from build123d import *

# Parameters (mm, degrees)
F0_R      = 15.4644174612
F1_DEPTH  = 7.5
F3_DEPTH  = 3.5
F5_DEPTH  = 7.5
F7_DEPTH  = 7.5
F9_DEPTH  = 7.5
F11_DEPTH = 7.5
F13_DEPTH = 7.5
F15_DEPTH = 7.5
F17_DEPTH = 7.5
F18_W     = 5.4945703596
F18_H     = 28.8444776088
F19_DEPTH = 7.5
F22_DEPTH = 7.5


with BuildPart() as f1:
    # F0 (on Front) → F1 (new body)
    with BuildSketch(Plane.XZ):
        Circle(F0_R)
    extrude(amount=-F1_DEPTH)

    # F2 (on Front) → F3 (join)
    with BuildSketch(Plane.XZ):
        Polygon((3.5883630626, 11.3469837233), (-3.3943967428, 11.3469837233), (-3.3943967428, 3.5883623641), (-10.7650868595, 3.5883623641), (-10.7650868595, -3.5883623641), (-3.3943967428, -3.5883623641), (-3.3943967428, -11.9288796559), (3.5883630626, -11.9288796559), (3.5883630626, -3.5883623641), (11.5409484133, -3.5883623641), (11.5409484133, 3.5883623641), (3.5883630626, 3.5883623641), align=None)
    extrude(amount=F3_DEPTH)

    # F4 (on face) → F5 (join)
    with BuildSketch(Plane.XZ):
        with BuildLine():
            Line((-40.2478465542, -5.0589637569), (-14.6135243224, -5.0589637569))
            ThreePointArc((-14.6135243224, -5.0589637569), (-15.4624028659, 0.2496097512), (-14.442618561, 5.5280174129))
            Line((-14.442618561, 5.5280174129), (-40.2478465542, 5.5280174129))
            Line((-40.2478465542, 5.5280174129), (-40.2478465542, -5.0589637569))
        make_face()
    extrude(amount=-F5_DEPTH)

    # F6 (on face) → F7 (join)
    with BuildSketch(Plane.XZ):
        with BuildLine():
            Line((39.8599132895, 5.5280174129), (14.442618561, 5.5280174129))
            ThreePointArc((14.442618561, 5.5280174129), (15.4559066, 0.512989853), (14.7773852023, -4.5581897721))
            Line((14.7773852023, -4.5581897721), (39.8599132895, -4.5581897721))
            Line((39.8599132895, -4.5581897721), (39.8599132895, 5.5280174129))
        make_face()
    extrude(amount=-F7_DEPTH)

    # F8 (on face) → F9 (join)
    with BuildSketch(Plane.XZ):
        with BuildLine():
            ThreePointArc((13.3392752441, -7.8238061951), (-0.2412620254, -15.4625353694), (-13.5768721894, -7.4038333969))
            Line((-13.5768721894, -7.4038333969), (0, -38.1142273545))
            Line((0, -38.1142273545), (13.3392752441, -7.8238061951))
        make_face()
    extrude(amount=-F9_DEPTH)

    # F10 (on face) → F11 (join)
    with BuildSketch(Plane.XZ):
        with BuildLine():
            Line((1.4583327306, 20.6556674093), (-1.6825530911, 20.6556674093))
            Line((-1.6825530911, 20.6556674093), (-1.6825530911, 15.3955017152))
            Line((-1.6825530911, 15.3955017152), (-1.4583327306, 15.3955017152))
            ThreePointArc((-1.4583327306, 15.3955017152), (0, 15.4644174612), (1.4583327306, 15.3955017152))
            Line((1.4583327306, 15.3955017152), (1.4583327306, 20.6556674093))
        make_face()
    extrude(amount=-F11_DEPTH)

    # F12 (on face) → F13 (join)
    with BuildSketch(Plane.XZ):
        with BuildLine():
            ThreePointArc((1.4583327306, 15.4214656697), (4.3270974304, 17.3693579241), (5.4335625702, 20.6556674093))
            ThreePointArc((5.4335625702, 20.6556674093), (-3.1922832508, 25.05259018), (-1.6825530911, 15.4891775661))
            Line((-1.6825530911, 15.4891775661), (-1.6825530911, 20.6556674093))
            Line((-1.6825530911, 20.6556674093), (1.4583327306, 20.6556674093))
            Line((1.4583327306, 20.6556674093), (1.4583327306, 15.4214656697))
        make_face()
    extrude(amount=-F13_DEPTH)

    # F14 (on face) → F15 (join)
    with BuildSketch(Plane.XZ):
        with BuildLine():
            Line((35.3987067938, 27.0581915975), (2.0601032187, 15.6277874452))
            ThreePointArc((2.0601032187, 15.6277874452), (1.7622400662, 15.5158121435), (1.4583327306, 15.4214656697))
            Line((1.4583327306, 15.4214656697), (1.4583327306, 15.3955017152))
            ThreePointArc((1.4583327306, 15.3955017152), (9.3569158706, 12.312446256), (14.442618561, 5.5280174129))
            Line((14.442618561, 5.5280174129), (35.3987067938, 27.0581915975))
        make_face()
    extrude(amount=-F15_DEPTH)

    # F16 (on face) → F17 (join)
    with BuildSketch(Plane.XZ):
        with BuildLine():
            Line((-1.6825530911, 15.3955017152), (-1.6825530911, 15.4891775661))
            Line((-1.6825530911, 15.4891775661), (-33.5039995381, 25.8523592827))
            Line((-33.5039995381, 25.8523592827), (-14.442618561, 5.5280174129))
            ThreePointArc((-14.442618561, 5.5280174129), (-9.3569158706, 12.312446256), (-1.4583327306, 15.3955017152))
            Line((-1.4583327306, 15.3955017152), (-1.6825530911, 15.3955017152))
        make_face()
    extrude(amount=-F17_DEPTH)

    # F21 (on face) → F22 (join)
    with BuildSketch(Plane.XZ):
        with BuildLine():
            Line((-2.9614820185, 49.562137616), (-2.9614820185, 25.2112383349))
            ThreePointArc((-2.9614820185, 25.2112383349), (-0.8941182921, 26.0151594267), (1.3222555048, 25.9258896612))
            Line((1.3222555048, 25.9258896612), (2.0601032187, 26.0489840022))
            Line((2.0601032187, 26.0489840022), (2.0601032187, 49.562137616))
            Line((2.0601032187, 49.562137616), (-2.9614820185, 49.562137616))
        make_face()
    extrude(amount=-F22_DEPTH)


with BuildPart() as f19:
    # F18 (on Front) → F19 (new body)
    with BuildSketch(Plane.XZ):
        with Locations((0.3433788661, 40.6340872869)):
            Rectangle(F18_W, F18_H)
    extrude(amount=-F19_DEPTH)


solid = f1.part
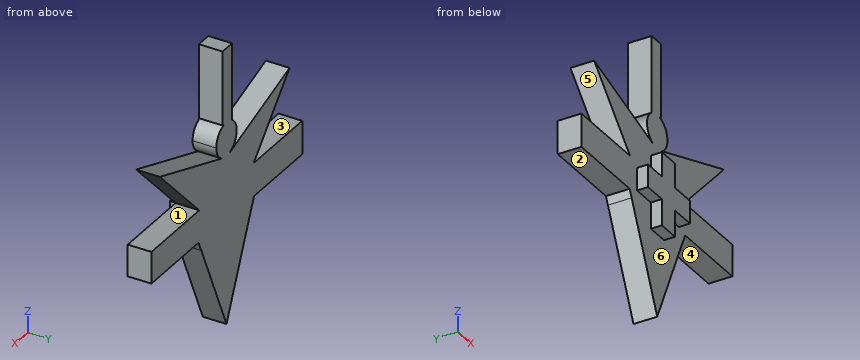
For this review, take the finished solid that the model builds, in its own axes (mm). Face numbers are marked on the shaded views. A direction names the side the tool comes from. Coordinates: 2 decimals unless noted, no trailing zeros. Order: outer loops, then holes, each group sorted by start corner. A loop starts at its lowest first (then second) coordinate and runs counter-clockwise, first axis right, second up. Notation, with made-up numbers: (18, 66.25) - (47, 66.25) arc R8 cw to (47, 81.25) - close; hole circle Ø2 at (-30.75, 45). An arc over 180 degrees is marked (long way). Answer as CSV lines item,"result". Start each with the question number.
1) Add section A-A (x = -16). State the section outline as (y, z) points.
2) Add section B-B (y = 3.25). State the section outline as (x, z) points.
3) Add section D-D (x = 6.5). State the section outline as (y, z) points, then the cut area to 3 significant figures.
4) Insertion check: P1, Ø1, axis at x = 1.5, y = -1.5, coming from the +Z side; P2, Ø1.8, axis at y = -2, z = 1, coming from the -X side; P3, Ø2, axis at y = 4, z = 38, coming from the +X side. Each pin has a flat end and moves straight along its axis. Give the tip position at first contact, or say it passes through.
5) To check wall thickness, follow line 1 along Z through (x, y) = (-4.5, -0.5); line 2 along Y through (x, z) = (12.5, 18); line 3 along Z through (x, y) = (-26.5, 2). State the ranges of each line that lie inside material, in increasing order. Write a range as [from, to].
6) Draft analysis for pull direction Z (two halves, no side actions). For the marked faces 4, 5 and 6, state which applies: +Z half, -Z half, draft (parallel to the pull), parting line (faces both ways), or undercut.
7) Add section C-C (z = 0). State the section outline as (x, y) points.
8) Machinability: for the marked faces 1, 2 and 3, which of the approach directions +Z, -Z, +X, -X, +Y, -Y give a long, thin tool a straight path to every point of the face, cutting with its end or side? Answer none if there is none.
Result:
1,outline,"(0, -5.06) - (7.5, -5.06) - (7.5, 5.53) - (0, 5.53) - close; (0, 7.19) - (7.5, 7.19) - (7.5, 20.15) - (0, 20.15) - close"
2,outline,"(-40.25, -5.06) - (-14.61, -5.06) arc R15.46 ccw to (-13.58, -7.4) - (0, -38.11) - (13.34, -7.82) arc R15.46 ccw to (14.78, -4.56) - (39.86, -4.56) - (39.86, 5.53) - (14.44, 5.53) - (35.4, 27.06) - (2.06, 15.63) arc R5.43 ccw to (1.32, 25.93) - (2.06, 26.05) - (2.06, 49.56) - (-2.96, 49.56) - (-2.96, 25.21) arc R5.43 ccw to (-1.68, 15.49) - (-33.5, 25.85) - (-14.44, 5.53) - (-40.25, 5.53) - close"
3,outline,"(-3.5, -3.59) - (0, -3.59) - (0, -23.35) - (7.5, -23.35) - (7.5, 17.15) - (0, 17.15) - (0, 3.59) - (-3.5, 3.59) - close"
3,area,"329 mm^2"
4,P1,"z = 11.35"
4,P2,"x = -10.77"
4,P3,"x = 2.06"
5,line 1,"[-3.59, 3.59]"
5,line 2,"[0, 7.5]"
5,line 3,"[-5.06, 5.53], [18.38, 23.57]"
6,face 4,"-Z half"
6,face 5,"undercut"
6,face 6,"draft"
7,outline,"(-40.25, 0) - (-10.77, 0) - (-10.77, -3.5) - (11.54, -3.5) - (11.54, 0) - (39.86, 0) - (39.86, 7.5) - (-40.25, 7.5) - close"
8,face 1,"+X, +Y, -Y"
8,face 2,"-Z, -X, +Y, -Y"
8,face 3,"-X, +Y, -Y"
